Work out the finished part from the listing and answer in its coordinate system (mm). Give positions to 0.01 mm unless a question says otherwise; leave off trailing zeros. Loops run counter-clockwise (first coordinate to the right, second up) from the corner with the lowest first, then second, coordinate; pieces in that order, holes last.
from build123d import *

# Parameters (mm, degrees)
SKETCH1_W           = 190
SKETCH1_H           = 165
SKETCH1_W_2         = 80
SKETCH1_H_2         = 42.5
BOSS_EXTRUDE1_DEPTH = 6
CUT_EXTRUDE1_DEPTH  = 15
CUT_EXTRUDE2_DEPTH  = 15


with BuildPart() as part:
    # Sketch1 → Boss-Extrude1 (new body)
    with BuildSketch(Plane(origin=(0, 0, 0), x_dir=(1, 0, 0), z_dir=(0, 1, 0))):
        Rectangle(SKETCH1_W, SKETCH1_H)
        with Locations((45, 15.25)):
            Rectangle(SKETCH1_W_2, SKETCH1_H_2, mode=Mode.SUBTRACT)
        with Locations((-45, 15.25)):
            Rectangle(SKETCH1_W_2, SKETCH1_H_2, mode=Mode.SUBTRACT)
    extrude(amount=BOSS_EXTRUDE1_DEPTH)

    # Sketch2 → Cut-Extrude1 (cut)
    with BuildSketch(Plane.ZY.offset(-85)):
        Polygon((-43.650521556, 6), (-36.5, 0), (-36.5, 6), align=None)
    extrude(amount=CUT_EXTRUDE1_DEPTH, mode=Mode.SUBTRACT)

    # Sketch3 → Cut-Extrude2 (cut)
    with BuildSketch(Plane(origin=(-85, 0, 0), x_dir=(0, 0, -1), z_dir=(1, 0, 0))):
        Polygon((-6, 0), (-13.150521556, 6), (-6, 6), align=None)
    extrude(amount=CUT_EXTRUDE2_DEPTH, mode=Mode.SUBTRACT)


solid = part.part
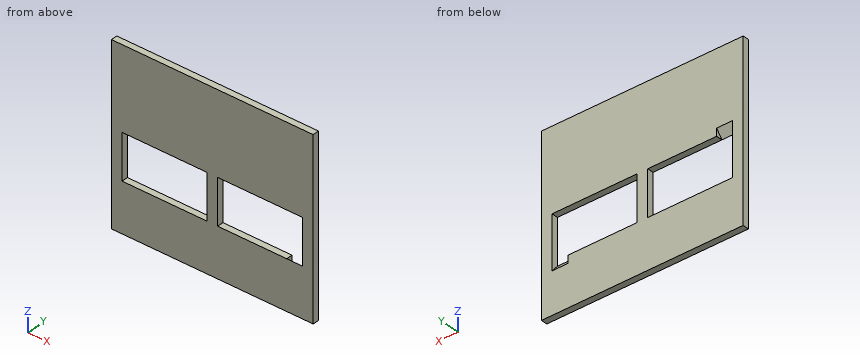
Item 1: Find section A-A, the plane z = -30.5. Write down the section's boundary in (x, y), plus the area to 3 significant figures.
Item 2: Find section D-D, the plane x = 80. Write down the section's boundary in (y, z).
Item 3: Consider line 1 (X direction, y = 3.25, z = 4); line 2 (Z direction, x = 13.5, y = 4.5); line 3 (Z direction, x = -77, y = 4.75). Determine where each line is inside the solid, lowest interval first.
Item 4: Find section B-B, the plane x = -27. Write down the section's boundary in (y, z).
Item 5: Find section C-C, the plane y = 1. Write down the section's boundary in (x, z).
Ans:
1. outline: (-95, 0) - (-85, 0) - (-85, 6) - (-95, 6) - close; (-5, 0) - (5, 0) - (5, 6) - (-5, 6) - close; (85, 0) - (95, 0) - (95, 6) - (85, 6) - close
1. area: 180 mm2
2. outline: (0, -82.5) - (6, -82.5) - (6, -43.65) - (0, -36.5) - close; (0, 6) - (6, 6) - (6, 82.5) - (0, 82.5) - close
3. line 1: x = -95 to -85, -5 to 5, 85 to 95
3. line 2: z = -82.5 to -36.5, 6 to 82.5
3. line 3: z = -82.5 to -36.5, 11.66 to 82.5
4. outline: (0, -82.5) - (6, -82.5) - (6, -36.5) - (0, -36.5) - close; (0, 6) - (6, 6) - (6, 82.5) - (0, 82.5) - close
5. outline: (-95, -82.5) - (95, -82.5) - (95, 82.5) - (-95, 82.5) - close; hole (-85, -36.5) - (-5, -36.5) - (-5, 6) - (-70, 6) - (-70, 7.19) - (-85, 7.19) - close; hole (5, -36.5) - (70, -36.5) - (70, -37.69) - (85, -37.69) - (85, 6) - (5, 6) - close
